The model under review builds one solid part; all positions refer to its coordinate system, in mm. Give positions to 0.01 mm unless a question says otherwise; leave off trailing zeros. Write each loop counter-clockwise with the first axis right and the second up, starting at its lowest first coordinate (ties: lowest second). Pieces come first, ordered by that corner, then holes.
Autodesk Inventor part; units mm, degrees
ref_plane "YZ Plane" through (0, 0, 0) normal (1, 0, 0) x (0, 1, 0)
ref_plane "XZ Plane" through (0, 0, 0) normal (0, 1, 0) x (-1, 0, 0)
ref_plane "XY Plane" through (0, 0, 0) normal (0, 0, 1) x (1, 0, 0)
sketch "Boceto1" plane through (0, 0, 0) normal (0, 0, 1) x (1, 0, 0)
  line L0 (0, 0) -> (0, 210)
  line L1 (0, 210) -> (450, 210)
  line L2 (450, 210) -> (450, 0)
  line L3 (450, 0) -> (0, 0)
  line L4 (0, 210) -> (5, 210)
  line L5 (5, 205) -> (50, 205)
  line L6 (50, 205) -> (50, 202)
  line L7 (5, 205) -> (5, 174.29)
  line L8 (5, 174.29) -> (8, 174.29)
  line L9 (8, 174.29) -> (8, 202)
  line L10 (8, 202) -> (50, 202)
  line L11 (0, 0) -> (5, 0)
  line L12 (0, 0) -> (5, 0)
  line L13 (5, 5) -> (50, 5)
  line L14 (5, 5) -> (5, 35.71)
  line L15 (5, 35.71) -> (8, 35.71)
  line L16 (50, 5) -> (50, 8)
  line L17 (8, 35.71) -> (8, 8)
  line L18 (8, 8) -> (50, 8)
  line L19 (450, 0) -> (445, 0)
  line L20 (445, 5) -> (445, 35.71)
  line L21 (445, 35.71) -> (442, 35.71)
  line L22 (445, 5) -> (400, 5)
  line L23 (400, 5) -> (400, 8)
  line L24 (400, 8) -> (442, 8)
  line L25 (442, 8) -> (442, 35.71)
  line L26 (450, 210) -> (445, 210)
  line L27 (445, 205) -> (400, 205)
  line L28 (445, 205) -> (445, 174.29)
  line L29 (445, 174.29) -> (442, 174.29)
  line L30 (400, 205) -> (400, 202)
  line L31 (400, 202) -> (442, 202)
  line L32 (442, 202) -> (442, 174.29)
  line L33 (5, 63.43) -> (5, 91.14)
  line L34 (5, 91.14) -> (8, 91.14)
  line L35 (8, 91.14) -> (8, 63.43)
  line L36 (8, 63.43) -> (5, 63.43)
  line L37 (5, 118.86) -> (5, 146.57)
  line L38 (5, 118.86) -> (8, 118.86)
  line L39 (8, 118.86) -> (8, 146.57)
  line L40 (8, 146.57) -> (5, 146.57)
  line L41 (445, 63.43) -> (445, 91.14)
  line L42 (445, 63.43) -> (442, 63.43)
  line L43 (442, 63.43) -> (442, 91.14)
  line L44 (442, 91.14) -> (445, 91.14)
  line L45 (445, 118.86) -> (442, 118.86)
  line L46 (442, 118.86) -> (442, 146.57)
  line L47 (442, 146.57) -> (445, 146.57)
  line L48 (445, 146.57) -> (445, 118.86)
  line L49 (350, 205) -> (300, 205)
  line L50 (300, 205) -> (300, 202)
  line L51 (300, 202) -> (350, 202)
  line L52 (350, 202) -> (350, 205)
  line L53 (250, 205) -> (200, 205)
  line L54 (200, 205) -> (200, 202)
  line L55 (200, 202) -> (250, 202)
  line L56 (250, 202) -> (250, 205)
  line L57 (150, 205) -> (100, 205)
  line L58 (100, 205) -> (100, 202)
  line L59 (100, 202) -> (150, 202)
  line L60 (150, 202) -> (150, 205)
  line L61 (350, 8) -> (300, 8)
  line L62 (300, 8) -> (300, 5)
  line L63 (300, 5) -> (350, 5)
  line L64 (350, 5) -> (350, 8)
  line L65 (250, 8) -> (200, 8)
  line L66 (200, 8) -> (200, 5)
  line L67 (200, 5) -> (250, 5)
  line L68 (250, 5) -> (250, 8)
  line L69 (150, 8) -> (100, 8)
  line L70 (100, 8) -> (100, 5)
  line L71 (100, 5) -> (150, 5)
  line L72 (150, 5) -> (150, 8)
  line L73 (450, 0) -> (450, 30)
  line L74 (380, 30) -> (380, 110)
  line L75 (380, 30) -> (370, 30)
  line L76 (370, 30) -> (370, 100)
  line L77 (380, 110) -> (280, 110)
  line L78 (370, 100) -> (280, 100)
  line L79 (280, 110) -> (280, 180)
  line L80 (280, 100) -> (280, 30)
  line L81 (280, 30) -> (270, 30)
  line L82 (270, 30) -> (270, 100)
  line L83 (280, 180) -> (270, 180)
  line L84 (270, 180) -> (270, 110)
  line L85 (270, 100) -> (180, 100)
  line L86 (270, 110) -> (180, 110)
  line L87 (180, 110) -> (180, 180)
  line L88 (180, 180) -> (170, 180)
  line L89 (170, 180) -> (170, 110)
  line L90 (180, 100) -> (180, 30)
  line L91 (180, 30) -> (170, 30)
  line L92 (170, 30) -> (170, 100)
  line L93 (170, 110) -> (80, 110)
  line L94 (80, 110) -> (80, 180)
  line L95 (80, 180) -> (70, 180)
  line L96 (70, 180) -> (70, 100)
  line L97 (70, 100) -> (170, 100)
  dimension "d93" = 450
  dimension "d94" = 210
  dimension "d95" = 210
  dimension "d96" = 450
  dimension "d97" = 5
  dimension "d98" = 30.71
  dimension "d99" = 45
  dimension "d100" = 5
  dimension "d101" = 3
  dimension "d102" = 3
  dimension "d103" = 5
  dimension "d104" = 5
  dimension "d105" = 3
  dimension "d106" = 30.71
  dimension "d107" = 45
  dimension "d108" = 3
  dimension "d109" = 5
  dimension "d110" = 30.71
  dimension "d111" = 45
  dimension "d112" = 5
  dimension "d113" = 3
  dimension "d114" = 3
  dimension "d115" = 30.71
  dimension "d116" = 5
  dimension "d117" = 45
  dimension "d118" = 5
  dimension "d119" = 3
  dimension "d120" = 3
  dimension "d121" = 3
  dimension "d122" = 3
  dimension "d123" = 3
  dimension "d124" = 5
  dimension "d125" = 5
  dimension "d126" = 5
  dimension "d127" = 5
  dimension "d128" = 5
  dimension "d129" = 5
  dimension "d130" = 27.72
  dimension "d131" = 27.71
  dimension "d132" = 27.71
  dimension "d133" = 27.72
  dimension "d134" = 27.72
  dimension "d135" = 50
  dimension "d136" = 50
  dimension "d137" = 50
  dimension "d138" = 50
  dimension "d139" = 50
  dimension "d140" = 50
  dimension "d141" = 50
extrude "Extrusión1" add sketch "Boceto1" along normal blind 3
properties part number "Frontal" material "Madera (nogal)"
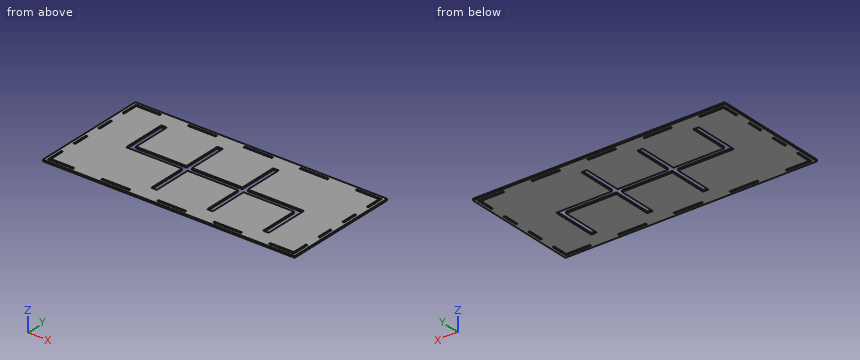
1) Consider section C-C, the plane x = 295.5. Give the boundary of the cut face in (y, z).
2) To check wall thickness, follow probe 1 along Y at (x, z) = (316, 2.2); probe 2 along X at (y, z) = (59, 2.25); probe 3 along X at (y, z) = (10.5, 1). State the ranges of each line that lie inside material, in increasing order.
3) Consider section D-D, the plane z = 2.3. State how many separate pieces and enclosed holes the cut face has, then the cut area to 3 significant figures.
4) Consider section A-A, the plane x = 344. Give the boundary of the cut face in (y, z), then the cut area to 3 significant figures.
5) Consider section B-B, the plane y = 158. Give the boundary of the cut face in (x, z).
Answer block:
1. outline: (0, 0) - (100, 0) - (100, 3) - (0, 3) - close; (110, 0) - (210, 0) - (210, 3) - (110, 3) - close
2. probe 1: y = 0 to 5, 8 to 100, 110 to 202, 205 to 210
2. probe 2: x = 0 to 170, 180 to 270, 280 to 370, 380 to 450
2. probe 3: x = 0 to 5, 8 to 442, 445 to 450
3. separate pieces: 1
3. enclosed holes: 15
3. area: 85,100 mm2
4. outline: (0, 0) - (5, 0) - (5, 3) - (0, 3) - close; (8, 0) - (100, 0) - (100, 3) - (8, 3) - close; (110, 0) - (202, 0) - (202, 3) - (110, 3) - close; (205, 0) - (210, 0) - (210, 3) - (205, 3) - close
4. area: 582 mm2
5. outline: (0, 0) - (70, 0) - (70, 3) - (0, 3) - close; (80, 0) - (170, 0) - (170, 3) - (80, 3) - close; (180, 0) - (270, 0) - (270, 3) - (180, 3) - close; (280, 0) - (450, 0) - (450, 3) - (280, 3) - close
